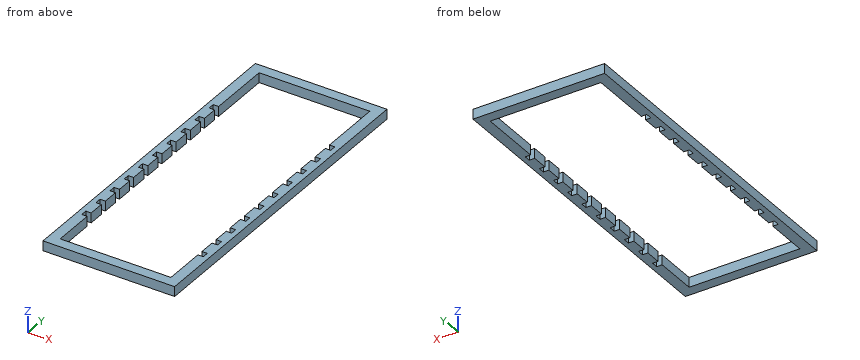
```python
from build123d import *

# Parameters (mm, degrees)
SKETCH1_W           = 67.31
SKETCH1_H           = 187.325
BOSS_EXTRUDE1_DEPTH = 5.9944
SKETCH2_W           = 6.604
SKETCH2_H           = 3.81
CUT_EXTRUDE1_DEPTH  = 6.9944


with BuildPart() as part:
    # Sketch1 → Boss-Extrude1 (new body)
    with BuildSketch(Plane.XY):
        Polygon((0, 0), (6.35, 0), (73.66, 0), (80.01, 0), (80.01, 200.025), (73.66, 200.025), (6.35, 200.025), (0, 200.025), align=None)
        with Locations((40.005, 100.0125)):
            Rectangle(SKETCH1_W, SKETCH1_H, mode=Mode.SUBTRACT)
    extrude(amount=-BOSS_EXTRUDE1_DEPTH)

    # Sketch2 → Cut-Extrude1 (cut, through all)
    with BuildSketch(Plane.XY):
        with Locations((6.35, 33.655)):
            Rectangle(SKETCH2_W, SKETCH2_H)
        with Locations((6.35, 46.99)):
            Rectangle(SKETCH2_W, SKETCH2_H)
        with Locations((73.66, 33.655)):
            Rectangle(SKETCH2_W, SKETCH2_H)
        with Locations((73.66, 46.99)):
            Rectangle(SKETCH2_W, SKETCH2_H)
        with Locations((6.35, 60.325)):
            Rectangle(SKETCH2_W, SKETCH2_H)
        with Locations((73.66, 60.325)):
            Rectangle(SKETCH2_W, SKETCH2_H)
        with Locations((6.35, 73.66)):
            Rectangle(SKETCH2_W, SKETCH2_H)
        with Locations((73.66, 73.66)):
            Rectangle(SKETCH2_W, SKETCH2_H)
        with Locations((6.35, 86.995)):
            Rectangle(SKETCH2_W, SKETCH2_H)
        with Locations((73.66, 86.995)):
            Rectangle(SKETCH2_W, SKETCH2_H)
        with Locations((6.35, 100.33)):
            Rectangle(SKETCH2_W, SKETCH2_H)
        with Locations((73.66, 100.33)):
            Rectangle(SKETCH2_W, SKETCH2_H)
        with Locations((6.35, 113.665)):
            Rectangle(SKETCH2_W, SKETCH2_H)
        with Locations((73.66, 113.665)):
            Rectangle(SKETCH2_W, SKETCH2_H)
        with Locations((6.35, 127)):
            Rectangle(SKETCH2_W, SKETCH2_H)
        with Locations((73.66, 127)):
            Rectangle(SKETCH2_W, SKETCH2_H)
        with Locations((6.35, 140.335)):
            Rectangle(SKETCH2_W, SKETCH2_H)
        with Locations((73.66, 140.335)):
            Rectangle(SKETCH2_W, SKETCH2_H)
        with Locations((6.35, 153.67)):
            Rectangle(SKETCH2_W, SKETCH2_H)
        with Locations((73.66, 153.67)):
            Rectangle(SKETCH2_W, SKETCH2_H)
    extrude(amount=-CUT_EXTRUDE1_DEPTH, mode=Mode.SUBTRACT)


solid = part.part
```
Read the model definition and answer for the solid it produces. Units are mm, in the model's axes. Coordinates: 2 decimals unless noted, no trailing zeros. Loops run counter-clockwise (first coordinate to the right, second up) from the corner with the lowest first, then second, coordinate; pieces in that order, holes last. Notation, with made-up numbers: (82, 39) - (108, 39) arc R21 cw to (108, 56) - close; hole circle Ø11 at (57.25, 68.25). An arc over 180 degrees is marked (long way). Answer in a Markdown table with one row per item.
1. Given pin 1 (1.7 mm diameter, centred on x = 74.5, z = -3, fed in from -Y), flat-ended and moving along its own axis, determine where the tip first touches the part or whether it passes through.
Conclusion:
| item | result |
|---|---|
| pin 1 | stops at y = 0 |
2. Find section A-A, the plane y = 39.5. Write down the section's boundary in (x, z), then the cut area to 3 significant figures.
Conclusion:
| item | result |
|---|---|
| outline | (0, -5.99) - (6.35, -5.99) - (6.35, 0) - (0, 0) - close; (73.66, -5.99) - (80.01, -5.99) - (80.01, 0) - (73.66, 0) - close |
| area | 76.1 mm² |
3. Straight lines are drawn through the part: line 1 (X direction, y = 84, z = -3.15); line 2 (Y direction, x = 66, z = -2.9) (3 decimals); line 3 (X direction, y = 112, z = -0.25). For each, find the intervals that lie inside material, in ascending order.
Conclusion:
| item | result |
|---|---|
| line 1 | x = 0 to 6.35, 73.66 to 80.01 |
| line 2 | y = 0 to 6.35, 193.675 to 200.025 |
| line 3 | x = 0 to 3.05, 76.96 to 80.01 |
4. Find section B-B, the plane x = 52.5. Write down the section's boundary in (y, z) (3 decimals).
Conclusion:
| item | result |
|---|---|
| outline | (0, -5.994) - (6.35, -5.994) - (6.35, 0) - (0, 0) - close; (193.675, -5.994) - (200.025, -5.994) - (200.025, 0) - (193.675, 0) - close |
